Verification items for the finished model (mm, model axes). Face numbers are marked on the shaded views. A direction names the side the tool comes from. Give positions to 0.01 mm unless a question says otherwise; leave off trailing zeros. Write each loop counter-clockwise with the first axis right and the second up, starting at its lowest first coordinate (ties: lowest second). Pieces come first, ordered by that corner, then holes. Notation, with made-up numbers: (85.5, 25.5) - (103.5, 25.5) arc R17 ccw to (103.5, 34.5) - close; hole circle Ø3 at (78, -22.75). An arc over 180 degrees is marked (long way). Answer as a JSON object with one key per item and string values. Group by question number.
Item 1: Sectioned sample at C-C, the plane y = -4.5. Count the separate pieces of the cut face and the enclosed holes in it, and give its area (3 significant figures).
Item 2: Scan lines: line 1 along Z through (x, y) = (67, -4); line 2 along X through (y, z) = (-5.5, 11) (3 decimals); line 3 along X through (y, z) = (-6.5, 1) (3 decimals). Record each from-to range of solid material in increasing order. Write a range as [from, to].
Item 3: Sectioned sample at D-D, the plane x = 73. Record the boundary of the cut face in (y, z).
Item 4: Go/stop test with flat-tipped pins: pin 1 (11 mm diameter, centred on x = 67.5, z = 31, fed in from -Y); pin 2 (3 mm diameter, centred on y = -5, z = 50.5, fed in from -X) (3 decimals); pin 3 (6 mm diameter, centred on y = -6, z = 2.5, fed in from +X). Record where each tip stops, or that it passes through.
Item 5: Sectioned sample at B-B, the plane x = 37. Record the boundary of the cut face in (y, z).
Item 6: Draft check along Z on the marked faces 6, 7, 8 and 9. Enter one of: +Z half, -Z half, draft (parallel to the pull), parting line (faces both ways), or undercut.
Item 7: Tool access check on the marked faces 1, 2, 3, 4 and 5. Record the directions out of +Z, -Z, +X, -X, +Y, -Y that give a thin tool (end or side, any length) a straight path to the whole face; none if there is none.
Item 8: Sectioned sample at A-A, the plane z = 54.5. Record the boundary of the cut face in (x, y) (3 decimals), and give its area (3 significant figures).
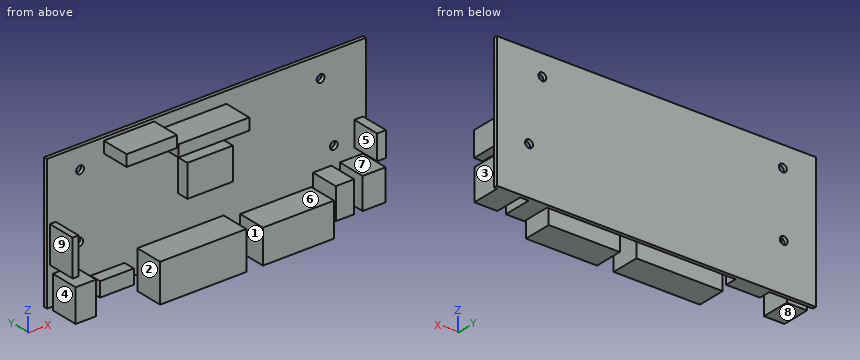
```python
from build123d import *

# Parameters (mm, degrees)
F0_W     = 139.065
F0_H     = 58.039
F0_R     = 1.7145
F1_DEPTH = 1.6002
F2_W     = 8.001
F2_H     = 13.589
F2_W_2   = 10.033
F2_W_3   = 30.861
F2_H_2   = 5.08
F2_W_4   = 21.971
F2_H_3   = 4.953
F2_W_5   = 2.54
F2_H_4   = 15.875
F2_W_6   = 37.592
F2_H_5   = 6.477
F2_W_7   = 30.988
F2_W_8   = 3.81
F2_H_6   = 10.795
F2_H_7   = 10.16
F2_H_8   = 8.255
F2_W_9   = 8.89
F2_H_9   = 1.524
F2_H_10  = 12.7
F3_DEPTH = 12.446
F2_W_10  = 19.812
F2_H_11  = 13.97
F2_W_11  = 14.732
F2_H_12  = 6.35
F4_DEPTH = 5.08


with BuildPart() as f1:
    # F0 (on Front) → F1 (new body)
    with BuildSketch(Plane.XZ):
        with Locations((69.5325, 29.0195)):
            Rectangle(F0_W, F0_H)
        with Locations((14.0462, 21.0058)):
            Circle(F0_R, mode=Mode.SUBTRACT)
        with Locations((125.0315, 21.0185)):
            Circle(F0_R, mode=Mode.SUBTRACT)
        with Locations((14.4145, 48.9585)):
            Circle(F0_R, mode=Mode.SUBTRACT)
        with Locations((119.2403, 48.9458)):
            Circle(F0_R, mode=Mode.SUBTRACT)
    extrude(amount=F1_DEPTH)

    # F2 (on face) → F3 (join)
    with BuildSketch(Plane.XZ.offset(1.6002)):
        with Locations((119.9515, 6.7945)):
            Rectangle(F2_W, F2_H)
        with Locations((132.6515, 6.7945)):
            Rectangle(F2_W_2, F2_H)
        with Locations((62.8015, 50.419)):
            Rectangle(F2_W_3, F2_H_2)
        with Locations((35.7505, 54.2925)):
            Rectangle(F2_W_4, F2_H_3)
        with Locations((2.54, 24.4475)):
            Rectangle(F2_W_5, F2_H_4)
        with Locations((58.166, -3.2385)):
            Rectangle(F2_W_6, F2_H_5)
        with Locations((99.695, -3.2385)):
            Rectangle(F2_W_7, F2_H_5)
        with Locations((135.89, 22.5425)):
            Rectangle(F2_W_8, F2_H_6)
        with Locations((58.166, 5.08)):
            Rectangle(F2_W_6, F2_H_7)
        with Locations((99.695, 4.1275)):
            Rectangle(F2_W_7, F2_H_8)
        with Locations((6.985, -0.762)):
            Rectangle(F2_W_9, F2_H_9)
        with Locations((6.985, 6.35)):
            Rectangle(F2_W_9, F2_H_10)
    extrude(amount=F3_DEPTH)

    # F2 (on face) → F4 (join)
    with BuildSketch(Plane.XZ.offset(1.6002)):
        with Locations((67.056, 32.385)):
            Rectangle(F2_W_10, F2_H_11)
        with Locations((26.416, 3.175)):
            Rectangle(F2_W_11, F2_H_12)
    extrude(amount=F4_DEPTH)


solid = f1.part
```
Geometry check:
{
 "1": {"separate pieces": "11", "enclosed holes": "0", "area": "2,170 mm^2"},
 "2": {"line 1": "[-6.48, 10.16], [25.4, 39.37], [47.88, 52.96]", "line 2": "[2.54, 11.43], [115.951, 123.952], [127.635, 137.668]", "line 3": "[2.54, 11.43], [19.05, 33.782], [39.37, 76.962], [84.201, 115.189], [115.951, 123.952], [127.635, 137.668]"},
 "3": {"outline": "(-14.05, -6.48) - (-1.6, -6.48) - (-1.6, 0) - (0, 0) - (0, 58.04) - (-1.6, 58.04) - (-1.6, 52.96) - (-14.05, 52.96) - (-14.05, 47.88) - (-1.6, 47.88) - (-1.6, 39.37) - (-6.68, 39.37) - (-6.68, 25.4) - (-1.6, 25.4) - (-1.6, 10.16) - (-14.05, 10.16) - close"},
 "4": {"pin 1": "y = -6.68", "pin 2": "x = 24.765", "pin 3": "x = 137.67"},
 "5": {"outline": "(-14.05, 51.82) - (-1.6, 51.82) - (-1.6, 0) - (0, 0) - (0, 58.04) - (-1.6, 58.04) - (-1.6, 56.77) - (-14.05, 56.77) - close"},
 "6": {"face 6": "+Z half", "face 7": "undercut", "face 8": "-Z half", "face 9": "draft"},
 "7": {"face 1": "+Z, -Z, -Y", "face 2": "-Z, -Y", "face 3": "-Z, +X, -Y", "face 4": "-Z, -X, -Y", "face 5": "+Z, -Y"},
 "8": {"outline": "(0, -1.6) - (24.765, -1.6) - (24.765, -14.046) - (46.736, -14.046) - (46.736, -1.6) - (139.065, -1.6) - (139.065, 0) - (0, 0) - close", "area": "496 mm^2"}
}
